Design review of the part built by this model. Coordinates are the model's own, in mm. A direction names the side the tool comes from. Coordinates: 2 decimals unless noted, no trailing zeros. Loops run counter-clockwise (first coordinate to the right, second up) from the corner with the lowest first, then second, coordinate; pieces in that order, holes last. Notation, with made-up numbers: (-3, 83.5) - (42, 83.5) arc R11 cw to (42, 100.5) - close; hole circle Ø2 at (52.25, -25.75). An arc over 180 degrees is marked (long way). One line per question, with ' | ' between items.
from build123d import *

# Parameters (mm, degrees)
F0_W     = 80
F0_H     = 26
F0_R     = 1.85
F1_DEPTH = 25
F3_R     = 3.25
F3_R_2   = 1.85
F4_DEPTH = 18
F5_DEPTH = 100
F6_R     = 1.825
F7_DEPTH = 90


with BuildPart() as f1:
    # F0 (on Top) → F1 (new body)
    with BuildSketch(Plane.XY):
        Rectangle(F0_W, F0_H)
        with Locations((-32, -8)):
            Circle(F0_R, mode=Mode.SUBTRACT)
        with Locations((0, -8)):
            Circle(F0_R, mode=Mode.SUBTRACT)
        with Locations((32, -8)):
            Circle(F0_R, mode=Mode.SUBTRACT)
        with Locations((-32, 8)):
            Circle(F0_R, mode=Mode.SUBTRACT)
        with Locations((0, 8)):
            Circle(F0_R, mode=Mode.SUBTRACT)
        with Locations((32, 8)):
            Circle(F0_R, mode=Mode.SUBTRACT)
    extrude(amount=F1_DEPTH)

    # F3 (on face) → F4 (cut)
    with BuildSketch(Plane.XY.offset(25)):
        with Locations((-32, -8)):
            Circle(F3_R)
        with Locations((-32, -8)):
            Circle(F3_R_2, mode=Mode.SUBTRACT)
        with Locations((-32, 8)):
            Circle(F3_R)
        with Locations((-32, 8)):
            Circle(F3_R_2, mode=Mode.SUBTRACT)
        with Locations((0, 8)):
            Circle(F3_R)
        with Locations((0, 8)):
            Circle(F3_R_2, mode=Mode.SUBTRACT)
        with Locations((0, -8)):
            Circle(F3_R)
        with Locations((0, -8)):
            Circle(F3_R_2, mode=Mode.SUBTRACT)
        with Locations((32, 8)):
            Circle(F3_R)
        with Locations((32, 8)):
            Circle(F3_R_2, mode=Mode.SUBTRACT)
        with Locations((32, -8)):
            Circle(F3_R)
        with Locations((32, -8)):
            Circle(F3_R_2, mode=Mode.SUBTRACT)
    extrude(amount=-F4_DEPTH, mode=Mode.SUBTRACT)

    # F2 (on face) → F5 (cut)
    with BuildSketch(Plane.YZ.offset(40)):
        with BuildLine():
            Line((-13, 25), (-13, 18))
            ThreePointArc((-13, 18), (0, 12), (13, 18))
            Line((13, 18), (13, 25))
            Line((13, 25), (-13, 25))
        make_face()
    extrude(amount=-F5_DEPTH, mode=Mode.SUBTRACT)

    # F6 (on face) → F7 (cut)
    with BuildSketch(Plane(origin=(0, 13, 0), x_dir=(-1, 0, 0), z_dir=(0, 1, 0))):
        with Locations((-24, 5.2)):
            Circle(F6_R)
        with Locations((-8, 5.2)):
            Circle(F6_R)
    extrude(amount=-F7_DEPTH, mode=Mode.SUBTRACT)


solid = f1.part
Q1. Take a section at C-C (x = -32.5). Give the boundary of the cut face in (y, z).
Returned:
outline: (-13, 0) - (-9.78, 0) - (-9.78, 7) - (-11.21, 7) - (-11.21, 16.19) arc R17.08 cw to (-13, 18) - close; (-6.22, 0) - (6.22, 0) - (6.22, 7) - (4.79, 7) - (4.79, 12.68) arc R17.08 cw to (-4.79, 12.68) - (-4.79, 7) - (-6.22, 7) - close; (9.78, 0) - (13, 0) - (13, 18) arc R17.08 cw to (11.21, 16.19) - (11.21, 7) - (9.78, 7) - close
Q2. Draft analysis for pull direction Y (two halves, no side actions). For faces 1 (the flat face through (-1, -13, 9)), 2 (the cylindrical face through (31.295, -11.173, 10.663)), 3 (the flat face through (-1, 13, 9)), 4 (the cylindrical face through (9.45, 0.18, 4.09)), state which applies: +Y half, -Y half, draft (parallel to the pull), parting line (faces both ways), or undercut.
Returned:
face 1: -Y half | face 2: undercut | face 3: +Y half | face 4: draft
Q3. Tool access review of faces 5 (the cylindrical face through (-33.468, 6.874, 3.451)), 6 (the cylindrical face through (-0.423, 11.222, 10.653)): name each direction out of +Z, -Z, +X, -X, +Y, -Y from which nothing blocks a thin tool from reaching the whole face with its end or side.
Returned:
face 5: +Z, -Z | face 6: +Z
Q4. Take a section at D-D (x = 7). Give the boundary of the cut face in (y, z), plus the area to 3 significant figures.
Returned:
outline: (-13, 0) - (13, 0) - (13, 3.67) - (-13, 3.67) - close; (-13, 6.73) - (13, 6.73) - (13, 18) arc R17.08 cw to (-13, 18) - close | area: 280 mm²
Q5. Take a section at A-A (z = 5.2). State how many separate pieces and enclosed holes the cut face has, plus the area to 3 significant figures.
Returned:
separate pieces: 3 | enclosed holes: 6 | area: 1,830 mm²
Q6. For pin 1 (8.5 mm diameter, centred on x = 0, y = -8, fed in from +Z); pin 2 (7 mm diameter, centred on x = -1, y = -7.5, fed in from +Z); pin 3 (6 mm diameter, centred on x = 22, y = -5.5, fed in from +Z), all flat-tipped, find the tip position at first contact; note any pin that passes through.
Returned:
pin 1: stops at z = 17.18 | pin 2: stops at z = 16 | pin 3: stops at z = 14.26
Q7. To check wall thickness, follow line 1 along X through (y, z) = (-8, 12.25); line 2 along Y through (x, z) = (-32, 10.25); line 3 along Y through (x, z) = (1, 1). State the ranges of each line that lie inside material, in increasing order.
Returned:
line 1: x = -40 to -35.25, -28.75 to -3.25, 3.25 to 28.75, 35.25 to 40 | line 2: y = -13 to -11.25, -4.75 to 4.75, 11.25 to 13 | line 3: y = -13 to -9.56, -6.44 to 6.44, 9.56 to 13
